Can you work these out from the model? Positions are in its coordinate system, mm. A direction names the side the tool comes from. Give positions to 0.01 mm unless a question says otherwise; leave off trailing zeros. Loops run counter-clockwise (first coordinate to the right, second up) from the corner with the lowest first, then second, coordinate; pieces in that order, holes last. Notation, with made-up numbers: (72.5, -25.75) - (122.5, -25.75) arc R26 ccw to (122.5, 2.25) - close; hole circle Ø6 at (89, -5.5). An arc over 180 degrees is marked (long way). Use a Markdown table: item, result. Add a question column.
```python
from build123d import *

# Parameters (mm, degrees)
SKETCH1_W           = 76.5
SKETCH1_H           = 42.5
BOSS_EXTRUDE1_DEPTH = 3
BOSS_EXTRUDE2_DEPTH = 42.5
FILLET1_R           = 5
FILLET2_R           = 5
FILLET3_R           = 5
FILLET4_R           = 5


with BuildPart() as part:
    # Sketch1 → Boss-Extrude1 (new body)
    with BuildSketch(Plane(origin=(0, 0, 0), x_dir=(1, 0, 0), z_dir=(0, 1, 0))):
        with Locations((38.25, 21.25)):
            Rectangle(SKETCH1_W, SKETCH1_H)
    extrude(amount=BOSS_EXTRUDE1_DEPTH)

    # Sketch2 → Boss-Extrude2 (add)
    with BuildSketch(Plane.XY):
        Polygon((76.5, 3), (76.5, 0), (97.713203436, 21.213203436), (97.713203436, 28.213203436), (95.591883092, 28.213203436), (95.591883092, 22.091883092), align=None)
    extrude(amount=-BOSS_EXTRUDE2_DEPTH)

    # Fillet1
    fillet1_edges = [part.edges().sort_by_distance(p)[0] for p in [
        (97.713203436, 21.213203436, -21.25),
        (76.5, 0, -21.25),
    ]]
    fillet(fillet1_edges, radius=FILLET1_R)

    # Fillet2
    fillet2_edges = [part.edges().sort_by_distance(p)[0] for p in [
        (0, 1.5, -42.5),
        (0, 1.5, 0),
    ]]
    fillet(fillet2_edges, radius=FILLET2_R)

    # Fillet3
    fillet3_edges = [part.edges().sort_by_distance(p)[0] for p in [
        (96.652543264, 28.213203436, 0),
        (96.652543264, 28.213203436, -42.5),
    ]]
    fillet(fillet3_edges, radius=FILLET3_R)

    # Fillet4
    fillet4_edges = [part.edges().sort_by_distance(p)[0] for p in [
        (76.5, 3, -21.25),
    ]]
    fillet(fillet4_edges, radius=FILLET4_R)


solid = part.part
```
1. Suppose I cut it at C-C (x = 65). List the corners of the cut face in (y, z) for me.
2. Please list where these lines run through material, in increasing order: line 1 along X through (y, z) = (27, -40); line 2 along Y through (x, z) = (44.5, -5); line 3 along X through (y, z) = (16.5, -15). Write a range as [from, to].
3. Suppose I cut it at A-A (z = -6.5). List the corners of the cut face in (x, y) for me, and give its area (3 significant figures).
4. Suppose I cut it at B-B (y = 7.5). List the corners of the cut face in (x, z) for me, and give its area (4 significant figures).
5. Suppose I cut it at D-D (z = -40). List the corners of the cut face in (x, y) for me.
6. Will these pins go through, and if not, where does the flat tip stop? P1, Ø3, axis at y = 24, z = -29, coming from the -X side; P2, Ø2, axis at y = 4, z = -11, coming from the +X side; P3, Ø2, axis at y = 18.5, z = -34.5, coming from the -X side.
7. On a 3-axis mill with a long thin cutter (end or side, diameter ignored), from which of +Z, -Z, +X, -X, +Y, -Y can I reach the whole of each face in a straight line? I mean faces 1 (the face through (37, 3, -22)), 2 (the face through (55, 2, 0)). Say none if no direction works.
Results below:
| question | item | result |
|---|---|---|
| 1 | outline | (0, -42.5) - (3, -42.5) - (3, 0) - (0, 0) - close |
| 2 | line 1 | [95.59, 97.71] |
| 2 | line 2 | [0, 3] |
| 2 | line 3 | [90, 93] |
| 3 | outline | (0, 0) - (74.43, 0) arc R5 ccw to (77.96, 1.46) - (96.25, 19.75) arc R5 ccw to (97.71, 23.28) - (97.71, 28.21) - (95.59, 28.21) - (95.59, 22.09) - (77.96, 4.46) arc R5 cw to (74.43, 3) - (0, 3) - close |
| 3 | area | 303 mm² |
| 4 | outline | (81, -42.5) - (84, -42.5) - (84, 0) - (81, 0) - close |
| 4 | area | 127.5 mm² |
| 5 | outline | (0.67, 0) - (74.43, 0) arc R5 ccw to (77.96, 1.46) - (96.25, 19.75) arc R5 ccw to (97.71, 23.28) - (97.71, 27.54) - (95.59, 27.54) - (95.59, 22.09) - (77.96, 4.46) arc R5 cw to (74.43, 3) - (0.67, 3) - close |
| 6 | P1 | x = 95.59 |
| 6 | P2 | x = 81.5 |
| 6 | P3 | x = 91 |
| 7 | face 1 | +Z, -Z, -X, +Y |
| 7 | face 2 | +Z, +X, -X, +Y, -Y |
